Input: part model. Units: mm. Frame: model coordinates. A direction names the side the tool comes from. Round coordinates to 2 decimals unless told otherwise and drop trailing zeros. Loops run counter-clockwise (first coordinate to the right, second up) from the corner with the lowest first, then second, coordinate; pieces in that order, holes last. Notation, with made-up numbers: (1.5, 32) - (35.5, 32) arc R19 ccw to (35.5, 60) - close; hole circle Ø7 at (41.5, -3). An arc over 180 degrees is marked (long way). One line per question, with ' | ' between items. Start each with the question number.
Item 1: First-contact query: pin 1 (9.5 mm diameter, centred on x = -59.5, y = 2.5, fed in from -Z); pin 2 (3 mm diameter, centred on x = 16.5, y = 21, fed in from -Z); pin 3 (1.5 mm diameter, centred on x = 4.5, y = 4, fed in from +Z); pin 4 (0.6 mm diameter, centred on y = -10, z = 1, fed in from +X). Flat tips, straight axial feed; report the tip coordinate or a pass-through.
Item 2: Set-up query: faces 4 (the face through (37, 0, 2)), 5 (the face through (-63, 0, 4)), 6 (the face through (-78.235, 0.692, 11.972)). Return all of +Z, -Z, +X, -X, +Y, -Y with unobstructed straight access to the full face (end or side cutting, diameter ignored); none if empty.
Item 3: Draft query along X for faces 1 (the face through (-17, 0, 10)), 2 (the face through (-82.4, 19.7, 4.9)), 3 (the face through (-93.992, 0.693, 4.93)). Return one class per face: pulls with the +X half, pulls with the -X half, needs draft (parallel to the pull), parting line crosses it, or undercut.
Item 4: Section D-D, the plane x = -70. Return loops of the section in (y, z), plus the area to 3 significant figures.
Item 5: Section C-C, the plane z = 12.5. Return loops of the section in (x, y), plus the area to 3 significant figures.
Item 6: Material intervals for line 1 along Y through (x, z) = (-44.82, 2.25); line 2 along Y through (x, z) = (16.5, 7.25); line 3 along X through (y, z) = (16, 3.75), sorted ascending.
Item 7: Section B-B, the plane x = 40. Return loops of the section in (y, z), plus the area to 3 significant figures.
Item 8: Section A-A, the plane y = -10. Return loops of the section in (x, z).
```python
from build123d import *

# Parameters (mm, degrees)
F0_R     = 3
F0_R_2   = 15.75
F1_DEPTH = 10
F2_DEPTH = 14
F0_W     = 50
F0_H     = 63
F0_R_3   = 2
F3_DEPTH = 10
F4_DEPTH = 4
F5_DEPTH = 2


with BuildPart() as f1:
    # F0 (on Top) → F1 (new body)
    with BuildSketch(Plane.XY):
        with BuildLine():
            Line((-62.5, -31.5), (12.5, -31.5))
            Line((12.5, -31.5), (12.5, 31.5))
            Line((12.5, 31.5), (-62.5, 31.5))
            ThreePointArc((-62.5, 31.5), (-94, 0), (-62.5, -31.5))
        make_face()
        with Locations((-80.18, -17.68)):
            Circle(F0_R, mode=Mode.SUBTRACT)
        with Locations((-44.82, -17.68)):
            Circle(F0_R, mode=Mode.SUBTRACT)
        with Locations((-62.5, 0)):
            Circle(F0_R_2, mode=Mode.SUBTRACT)
        with Locations((-80.18, 17.68)):
            Circle(F0_R, mode=Mode.SUBTRACT)
        with Locations((-44.82, 17.68)):
            Circle(F0_R, mode=Mode.SUBTRACT)
    extrude(amount=F1_DEPTH)

    # F0 (on Top) → F2 (join)
    with BuildSketch(Plane.XY):
        with Locations((-62.5, 0)):
            Circle(F0_R_2)
    extrude(amount=F2_DEPTH)

    # F0 (on Top) → F3 (join)
    with BuildSketch(Plane.XY):
        with Locations((37.5, 0)):
            Rectangle(F0_W, F0_H)
        with Locations((16.5, -21)):
            Circle(F0_R_3, mode=Mode.SUBTRACT)
        with Locations((58.5, -21)):
            Circle(F0_R_3, mode=Mode.SUBTRACT)
        with Locations((16.5, 21)):
            Circle(F0_R_3, mode=Mode.SUBTRACT)
        with Locations((58.5, 21)):
            Circle(F0_R_3, mode=Mode.SUBTRACT)
    extrude(amount=F3_DEPTH)

    # F0 (on Top) → F4 (cut)
    with BuildSketch(Plane.XY):
        with Locations((-62.5, 0)):
            Circle(F0_R_2)
    extrude(amount=F4_DEPTH, mode=Mode.SUBTRACT)

    # F0 (on Top) → F5 (cut)
    with BuildSketch(Plane.XY):
        with Locations((37.5, 0)):
            Rectangle(F0_W, F0_H)
        with Locations((16.5, -21)):
            Circle(F0_R_3, mode=Mode.SUBTRACT)
        with Locations((58.5, -21)):
            Circle(F0_R_3, mode=Mode.SUBTRACT)
        with Locations((16.5, 21)):
            Circle(F0_R_3, mode=Mode.SUBTRACT)
        with Locations((58.5, 21)):
            Circle(F0_R_3, mode=Mode.SUBTRACT)
    extrude(amount=F5_DEPTH, mode=Mode.SUBTRACT)


solid = f1.part
```
Return value:
1) pin 1: z = 4 | pin 2: through | pin 3: z = 10 | pin 4: x = 12.5
2) face 4: -Z, +X, +Y, -Y | face 5: -Z | face 6: +Z
3) face 1: needs draft | face 2: undercut | face 3: pulls with the -X half
4) outline: (-30.59, 0) - (-13.85, 0) - (-13.85, 4) - (13.85, 4) - (13.85, 0) - (30.59, 0) - (30.59, 10) - (13.85, 10) - (13.85, 14) - (-13.85, 14) - (-13.85, 10) - (-30.59, 10) - close | area: 612 mm2
5) outline: circle Ø31.5 at (-62.5, 0) | area: 779 mm2
6) line 1: -31.5 to -20.68, -14.68 to 14.68, 20.68 to 31.5 | line 2: -31.5 to -23, -19 to 19, 23 to 31.5 | line 3: -89.63 to -82.67, -77.69 to -47.31, -42.33 to 62.5
7) outline: (-31.5, 2) - (31.5, 2) - (31.5, 10) - (-31.5, 10) - close | area: 504 mm2
8) outline: (-92.37, 0) - (-74.67, 0) - (-74.67, 4) - (-50.33, 4) - (-50.33, 0) - (12.5, 0) - (12.5, 2) - (62.5, 2) - (62.5, 10) - (-50.33, 10) - (-50.33, 14) - (-74.67, 14) - (-74.67, 10) - (-92.37, 10) - close
